Here's how the part is built. I have some questions about the finished solid (model axes, mm). A direction names the side the tool comes from. Give positions to 0.01 mm unless a question says otherwise; leave off trailing zeros. Order: outer loops, then holes, each group sorted by start corner. A loop starts at its lowest first (then second) coordinate and runs counter-clockwise, first axis right, second up. Notation, with made-up numbers: M 42,-3 L 75,-3 A20 cw 75,32 Z; hole C 23.25,52 d10. An arc over 180 degrees is marked long. Use one line per item in the form item = value.
from build123d import *

# Parameters (mm, degrees)
F0_R      = 60.3592367884
F1_DEPTH  = 36.576
F2_W      = 98.3545593917
F2_H      = 66.0087950528
F3_DEPTH  = 5.08
F4_R      = 50.7859823722
F5_DEPTH  = 63.754
F6_DEPTH  = 15.24
F8_DEPTH  = 26.924
F10_DEPTH = 61.722


with BuildPart() as f1:
    # F0 (on Top) → F1 (new body)
    with BuildSketch(Plane.XY):
        Circle(F0_R)
    extrude(amount=F1_DEPTH)

    # F2 (on Top) → F3 (join)
    with BuildSketch(Plane.XY):
        with Locations((0.1538116485, -68.1532975286)):
            Rectangle(F2_W, F2_H)
    extrude(amount=F3_DEPTH)

    # F4 (on face) → F5 (cut)
    with BuildSketch(Plane.XY.offset(36.576)):
        Circle(F4_R)
    extrude(amount=-F5_DEPTH, mode=Mode.SUBTRACT)

    # F6 (add): a face of the model
    f6_faces = [f1.faces().sort_by_distance(p)[0] for p in [
        (0.1538116485, -101.157695055, 2.54),
    ]]
    extrude(f6_faces, amount=F6_DEPTH)

    # F7 (on face) → F8 (join)
    with BuildSketch(Plane.XY.offset(5.08)):
        with BuildLine():
            Line((-3.9780647494, -60.2436316555), (-3.9780647494, -116.397695055))
            Line((-3.9780647494, -116.397695055), (3.7339403637, -116.397695055))
            Line((3.7339403637, -116.397695055), (3.7339403637, -60.2436316555))
            ThreePointArc((3.7339403637, -60.2436316555), (0, -60.3592367884), (-3.7339403636, -60.2436316555))
            Line((-3.7339403636, -60.2436316555), (-3.9780647494, -60.2436316555))
        make_face()
    extrude(amount=F8_DEPTH)

    # F9 (on face) → F10 (cut)
    with BuildSketch(Plane.YZ.offset(3.7339403637)):
        Polygon((-116.397695055, 32.004), (-116.397695055, 5.08), (-60.2436316555, 32.004), align=None)
    extrude(amount=-F10_DEPTH, mode=Mode.SUBTRACT)


solid = f1.part
Q1. On a 3-axis mill with a long thin cutter (end or side, diameter ignored), from which of +Z, -Z, +X, -X, +Y, -Y can I reach the whole of each face in a straight line? I mean faces 1 (the face through (49.331, -75, 3)), 2 (the face through (-27, -84, 5.08)), 3 (the face through (26, -84, 5.08)). Say none if no direction works.
Found:
face_1 = +Z, -Z, +X, -Y
face_2 = +Z, -X, -Y
face_3 = +Z, +X, -Y
Q2. I'm going to push flat-ended pins straight in: pin 1 Ø8 at (y, z) = (-63.5, 9) entering from -X; pin 2 Ø1 at (x, z) = (-14, 22.5) entering from +Y; pin 3 Ø13.5 at (x, y) = (-15, -70.5) entering from +Z; pin 4 Ø1.5 at (x, y) = (5.5, -70.5) entering from -Z. Where does each tip first touch, or does it pass through?
Found:
pin_1 = -49.02
pin_2 = 58.83
pin_3 = 5.08
pin_4 = 0
Q3. I want a section at A-A on y = 0. Write out the boundary of the cut face in (x, z).
Found:
outline = M -60.36,0 L -50.79,0 L -50.79,36.58 L -60.36,36.58 Z; M 50.79,0 L 60.36,0 L 60.36,36.58 L 50.79,36.58 Z
Q4. I want a section at B-B on x = 0. Write out the boundary of the cut face in (y, z), then the cut area to 3 significant figures.
Found:
outline = M -116.4,0 L -50.79,0 L -50.79,36.58 L -60.36,36.58 L -60.36,32 L -60.24,32 L -116.4,5.08 Z; M 50.79,0 L 60.36,0 L 60.36,36.58 L 50.79,36.58 Z
area = 1,740 mm²
Q5. I need wall thicknesses on L1, parallel to Y at x = 1, z = 5; L2, parallel to Z at x = 15.5, y = -81; L3, parallel to Y at x = 27.5, z = 2.5. Which ranges of each line are inside material? Lowest first, please.
Found:
L1 = -116.4 to -50.78, 50.78 to 60.35
L2 = 0 to 5.08
L3 = -116.4 to -42.7, 42.7 to 53.73
Q6. I want a section at D-D on x = 41. Write out the boundary of the cut face in (y, z), then the cut area to 3 significant figures.
Found:
outline = M -116.4,0 L -29.97,0 L -29.97,36.58 L -44.3,36.58 L -44.3,5.08 L -116.4,5.08 Z; M 29.97,0 L 44.3,0 L 44.3,36.58 L 29.97,36.58 Z
area = 1,410 mm²
Q7. Thinking about a two-plate mould opening in X: for faces 4 (the face through (-32, -40, 36.576)), 5 (the face through (-49.023, -75, 3)), 6 (the face through (-40.302, -30.902, 18.544)), which applies, +X half, -X half, draft (parallel to the pull), parting line (faces both ways), or undercut?
Found:
face_4 = draft
face_5 = -X half
face_6 = undercut
Q8. I want a section at C-C on z = 10. Write out the boundary of the cut face in (x, y), then the cut area to 3 significant figures.
Found:
outline = M -3.98,-106.14 L 3.73,-106.14 L 3.73,-60.24 A60.36 ccw long -3.73,-60.24 L -3.98,-60.24 Z; hole C 0,0 d101.57
area = 3,700 mm²
